The drawing under review shows one solid part. Ordinate dimensions are in mm from its lowest x, y, z. A direction names the side the tool comes from. Give positions to 0.01 mm unless a question says otherwise; leave off trailing zeros. Loops run counter-clockwise (first coordinate to the right, second up) from the corner with the lowest first, then second, coordinate; pieces in that order, holes last.
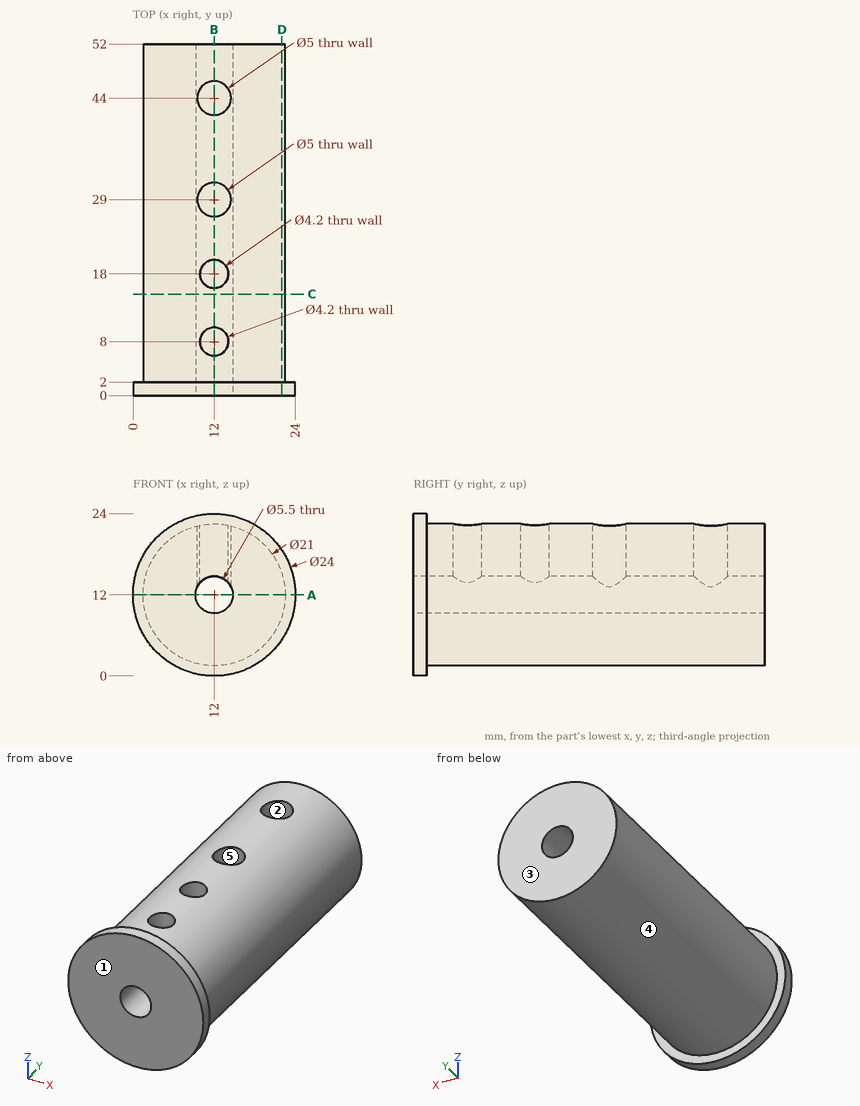
Item 1: For L1, parallel to Y at x = 12, z = 16.75; L2, parallel to X at y = 41.5, z = 12; L3, parallel to Z at x = 12, y = 20, list the stretches that pass through material, from the lowest coordinate up.
Answer:
L1: y = 0 to 5.9, 10.1 to 15.9, 20.1 to 26.5, 31.5 to 41.5, 46.5 to 52
L2: x = 1.5 to 9.25, 14.75 to 22.5
L3: z = 1.5 to 9.25
Item 2: Take a section at C-C on y = 15. Give the boundary of the cut face in (x, z).
Answer:
outline: circle Ø21 at (12, 12); hole circle Ø5.5 at (12, 12)
Item 3: Take a section at B-B on x = 12. Give the boundary of the cut face in (y, z), and give its area (3 significant figures).
Answer:
outline: (0, 0) - (2, 0) - (2, 1.5) - (52, 1.5) - (52, 9.25) - (0, 9.25) - close; (0, 14.75) - (5.9, 14.75) - (5.9, 22.5) - (2, 22.5) - (2, 24) - (0, 24) - close; (10.1, 14.75) - (15.9, 14.75) - (15.9, 22.5) - (10.1, 22.5) - close; (20.1, 14.75) - (26.5, 14.75) - (26.5, 22.5) - (20.1, 22.5) - close; (31.5, 14.75) - (41.5, 14.75) - (41.5, 22.5) - (31.5, 22.5) - close; (46.5, 14.75) - (52, 14.75) - (52, 22.5) - (46.5, 22.5) - close
area: 669 mm2
Item 4: Tool access review of the marked faces 1 and 2: name each direction out of +Z, -Z, +X, -X, +Y, -Y from which nothing blocks a thin tool from reaching the whole face with its end or side.
Answer:
face 1: +Z, -Z, +X, -X, -Y
face 2: +Z
Item 5: Clearance check with flat-ended pins moving along their axes: pin 1 Ø2 at (y, z) = (11.5, 16.5) entering from +X; pin 2 Ø6 at (y, z) = (20, 11) entering from -X; pin 3 Ø8 at (x, y) = (18.5, 16) entering from +Z; pin 4 Ø6.5 at (x, z) = (12, 12) entering from +Y. State where each tip first meets the part, or that it passes through.
Answer:
pin 1: stops at x = 21.9
pin 2: stops at x = 1.5
pin 3: stops at z = 22.2
pin 4: stops at y = 52
Item 6: Take a section at D-D on x = 22. Give the boundary of the cut face in (y, z).
Answer:
outline: (0, 5.37) - (2, 5.37) - (2, 8.8) - (52, 8.8) - (52, 15.2) - (2, 15.2) - (2, 18.63) - (0, 18.63) - close
Item 7: The part is to be moulded in two halves that separate along X. For the marked faces 3, 4 and 5, say which applies: released by +X, released by -X, zero draft, split by the parting line, or undercut.
Answer:
face 3: zero draft
face 4: split by the parting line
face 5: undercut
Item 8: Take a section at A-A on z = 12. Give the boundary of the cut face in (x, y).
Answer:
outline: (0, 0) - (9.25, 0) - (9.25, 52) - (1.5, 52) - (1.5, 2) - (0, 2) - close; (14.75, 0) - (24, 0) - (24, 2) - (22.5, 2) - (22.5, 52) - (14.75, 52) - close
